Could you check a few things on this model? Use its own coordinates, in mm. A direction names the side the tool comes from. Give positions to 0.01 mm unless a question says otherwise; leave off trailing zeros. Loops run counter-clockwise (first coordinate to the right, second up) from the corner with the lowest first, then second, coordinate; pieces in that order, holes last. Notation, with made-up numbers: (6, 64.5) -> (19, 64.5) arc R26 ccw to (19, 84.5) -> close; hole circle Ø1 at (57, 54.25). An arc over 180 degrees is marked (long way). Put each result on its own line as item: value.
```python
from build123d import *

# Parameters (mm, degrees)
CROQUIS2_R              = 3
SALIENTE_EXTRUIR2_DEPTH = 100
REDONDEO2_R             = 1


with BuildPart() as part:
    # Croquis2 → Saliente-Extruir2 (new body)
    with BuildSketch(Plane.XY):
        with BuildLine():
            Line((-10, 10), (-3, 10))
            Line((-3, 10), (-3, 8))
            Line((-3, 8), (-6.5, 8))
            Line((-6.5, 8), (-2.70506874, 4.20506874))
            ThreePointArc((-2.70506874, 4.20506874), (0, 5), (2.70506874, 4.20506874))
            Line((2.70506874, 4.20506874), (6.5, 8))
            Line((6.5, 8), (3, 8))
            Line((3, 8), (3, 10))
            Line((3, 10), (10, 10))
            Line((10, 10), (10, 3))
            Line((10, 3), (8, 3))
            Line((8, 3), (8, 6.5))
            Line((8, 6.5), (4.20506874, 2.70506874))
            ThreePointArc((4.20506874, 2.70506874), (5, 0), (4.20506874, -2.70506874))
            Line((4.20506874, -2.70506874), (8, -6.5))
            Line((8, -6.5), (8, -3))
            Line((8, -3), (10, -3))
            Line((10, -3), (10, -10))
            Line((10, -10), (3, -10))
            Line((3, -10), (3, -8))
            Line((3, -8), (6.5, -8))
            Line((6.5, -8), (2.70506874, -4.20506874))
            ThreePointArc((2.70506874, -4.20506874), (0, -5), (-2.70506874, -4.20506874))
            Line((-2.70506874, -4.20506874), (-6.5, -8))
            Line((-6.5, -8), (-3, -8))
            Line((-3, -8), (-3, -10))
            Line((-3, -10), (-10, -10))
            Line((-10, -10), (-10, -3))
            Line((-10, -3), (-8, -3))
            Line((-8, -3), (-8, -6.5))
            Line((-8, -6.5), (-4.20506874, -2.70506874))
            ThreePointArc((-4.20506874, -2.70506874), (-5, 0), (-4.20506874, 2.70506874))
            Line((-4.20506874, 2.70506874), (-8, 6.5))
            Line((-8, 6.5), (-8, 3))
            Line((-8, 3), (-10, 3))
            Line((-10, 3), (-10, 10))
        make_face()
        Circle(CROQUIS2_R, mode=Mode.SUBTRACT)
    extrude(amount=SALIENTE_EXTRUIR2_DEPTH)

    # Redondeo2
    redondeo2_edges = [part.edges().sort_by_distance(p)[0] for p in [
        (-10, 10, 50),
        (10, 10, 50),
        (10, -10, 50),
        (-10, -10, 50),
    ]]
    fillet(redondeo2_edges, radius=REDONDEO2_R)


solid = part.part
```
1. I'm going to push a flat-ended pin straight in: pin 1 (10 mm diameter, centred on x = 1.5, z = 64.5, fed in from -Y). Where does the tip first touch, or does it pass through?
Recorded:
pin 1: stops at y = -10
2. If we section it at A-A (x = 0): List the corners of the cut face in (y, z) for me.
Recorded:
outline: (-5, 0) -> (-3, 0) -> (-3, 100) -> (-5, 100) -> close; (3, 0) -> (5, 0) -> (5, 100) -> (3, 100) -> close
3. For faces 4 (the face through (9, 3, 49)), 5 (the face through (-3, 0, 49)), 6 (the face through (3, 9, 49)), which set-ups out of +Z, -Z, +X, -X, +Y, -Y let a thin tool reach every point of the face, with its end or its side?
Recorded:
face 4: +Z, -Z, +X
face 5: +Z, -Z
face 6: +Z, -Z, +Y
4. I need wall thicknesses on line 1 (Y direction, x = 0, z = 56); line 2 (Y direction, x = 8.5, z = 85); line 3 (X direction, y = -6, z = 95). Which ranges of each line are inside material? Lowest first, please.
Recorded:
line 1: y = -5 to -3, 3 to 5
line 2: y = -10 to -3, 3 to 10
line 3: x = -10 to -8, -7.5 to -4.5, 4.5 to 7.5, 8 to 10
5. Thinking about a two-plate mould opening in X: for faces 1 (the face through (-4.6, -6.1, 49.3)), 2 (the face through (-9, -3, 49)), 3 (the face through (-10, 6, 49)), which applies, pulls with the +X half, pulls with the -X half, needs draft (parallel to the pull), parting line crosses it, or undercut?
Recorded:
face 1: undercut
face 2: needs draft
face 3: pulls with the -X half
